```python
from build123d import *

# Parameters (mm, degrees)
F0_R     = 4.75
F0_W     = 3.6
F0_H     = 3.6
F1_DEPTH = 3.47
F2_R     = 4.75
F2_W     = 3.6
F2_H     = 3.6
F3_DEPTH = 1.5
F4_R     = 4.75
F4_R_2   = 3.75
F4_R_3   = 2.75
F4_R_4   = 1.75
F4_R_5   = 0.75
F5_DEPTH = 0.4
F6_R     = 0.4


with BuildPart() as f1:
    # F0 (on Top) → F1 (new body)
    with BuildSketch(Plane.XY):
        Circle(F0_R)
        Rectangle(F0_W, F0_H, mode=Mode.SUBTRACT)
    extrude(amount=F1_DEPTH)

    # F2 (on face) → F3 (join)
    with BuildSketch(Plane.XY.offset(3.47)):
        Circle(F2_R)
        Rectangle(F2_W, F2_H, mode=Mode.SUBTRACT)
        Rectangle(F2_W, F2_H)
    extrude(amount=F3_DEPTH)

    # F4 (on face) → F5 (join)
    with BuildSketch(Plane.XY.offset(4.97)):
        Circle(F4_R)
        Circle(F4_R_2, mode=Mode.SUBTRACT)
        Circle(F4_R_3)
        Circle(F4_R_4, mode=Mode.SUBTRACT)
        Circle(F4_R_5)
    extrude(amount=F5_DEPTH)

    # F6
    f6_edges = [f1.edges().sort_by_distance(p)[0] for p in [
        (-4.75, 0, 5.37),
        (-4.75, 0, 0),
    ]]
    fillet(f6_edges, radius=F6_R)


solid = f1.part
```
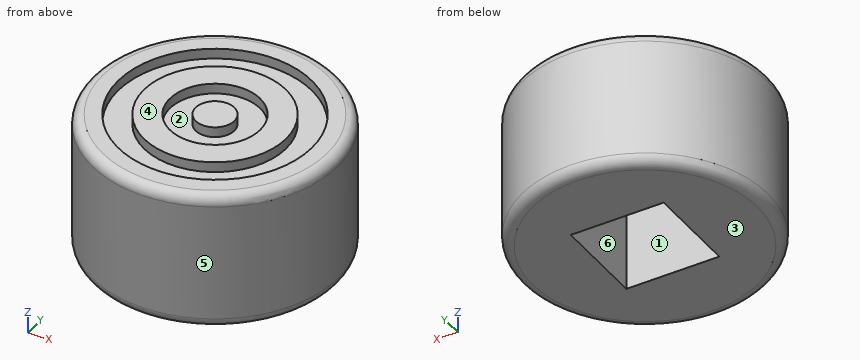
CAD build for the part. Positions are in the model's coordinates, mm. Face numbers are marked on the shaded views. A direction names the side the tool comes from. Coordinates: 2 decimals unless noted, no trailing zeros. Write each loop counter-clockwise with the first axis right and the second up, starting at its lowest first coordinate (ties: lowest second). Pieces come first, ordered by that corner, then holes.
(1) 3-axis set-ups, long thin cutter, end or side, ignore diameter. For the marked faces 1, 2 and 3: which of +Z, -Z, +X, -X, +Y, -Y reach the whole face in a straight line?
(2) Drill centre lines: probe 1 along X at (y, z) = (-1.5, 5); probe 2 along Y at (x, z) = (0, 5.3); probe 3 along Y at (x, z) = (0, 5.1). Where is each one in solid material? Low to high.
(3) Two-plate mould, pull along Y, no slides. Class the marked faces 4, 5 and 6: +Y half, -Y half, draft (parallel to the pull), parting line (faces both ways), or undercut.
(4) Cut at B-B, the plane y = 0. List the corners of the cut face in (x, z).
(5) Cut at A-A, the plane z = 2.05. List the corners of the cut face in (x, y), and give its area (3 significant figures).
(6) Flat gauge pins, fed straight in: pin 1 (5 mm diameter, centred on x = 3.5, y = 3.5, fed in from -Z); pin 2 (1.1 mm diameter, centred on x = 0, y = 0, fed in from -Z); pin 3 (2 mm diameter, centred on x = -2, z = 1, fed in from +Y); pin 4 (2 mm diameter, centred on x = -3, z = 2, fed in from -Y). Where does each tip first touch, or does it go through?
Geometry says:
1. face 1: -Z
1. face 2: +Z
1. face 3: -Z, +X, -X, +Y, -Y
2. probe 1: x = -4.51 to -3.44, -2.3 to -0.9, 0.9 to 2.3, 3.44 to 4.51
2. probe 2: y = -4.58 to -3.75, -2.75 to -1.75, -0.75 to 0.75, 1.75 to 2.75, 3.75 to 4.58
2. probe 3: y = -4.73 to -3.75, -2.75 to -1.75, -0.75 to 0.75, 1.75 to 2.75, 3.75 to 4.73
3. face 4: draft
3. face 5: parting line
3. face 6: undercut
4. outline: (-4.75, 0.4) arc R0.4 ccw to (-4.35, 0) - (-1.8, 0) - (-1.8, 3.47) - (1.8, 3.47) - (1.8, 0) - (4.35, 0) arc R0.4 ccw to (4.75, 0.4) - (4.75, 4.97) arc R0.4 ccw to (4.35, 5.37) - (3.75, 5.37) - (3.75, 4.97) - (2.75, 4.97) - (2.75, 5.37) - (1.75, 5.37) - (1.75, 4.97) - (0.75, 4.97) - (0.75, 5.37) - (-0.75, 5.37) - (-0.75, 4.97) - (-1.75, 4.97) - (-1.75, 5.37) - (-2.75, 5.37) - (-2.75, 4.97) - (-3.75, 4.97) - (-3.75, 5.37) - (-4.35, 5.37) arc R0.4 ccw to (-4.75, 4.97) - close
5. outline: circle Ø9.5 at (0, 0); hole (-1.8, -1.8) - (1.8, -1.8) - (1.8, 1.8) - (-1.8, 1.8) - close
5. area: 57.9 mm2
6. pin 1: stops at z = 0
6. pin 2: stops at z = 3.47
6. pin 3: stops at y = 4.64
6. pin 4: stops at y = -4.31
